The figure shows three views and two pictorial views of one solid part (mm, origin at its lowest corner). Answer the questions. A direction names the side the tool comes from. Give positions to 0.01 mm unless a question says otherwise; leave off trailing zeros. Loops run counter-clockwise (first coordinate to the right, second up) from the corner with the lowest first, then second, coordinate; pieces in that order, holes last. Notation, with made-up numbers: M -28,48 L 7,48 A35 ccw 7,87 Z; hole C 28.25,30.5 d10. An arc over 180 degrees is marked long. One line per item, written item: value. Start each with the question number.
Q1. The mould has two halves that part along Y. Classify the marked faces 1, 2 and 3: +Y half, -Y half, draft (parallel to the pull), parting line (faces both ways), or undercut.
Q2. A cutting plane is placed at A-A, the plane z = 8. Determine the outline of the cut face in (x, y), and give its area (4 significant figures).
Q3. A cutting plane is placed at D-D, the plane y = 13.25. Determine the outline of the cut face in (x, z).
Q4. A cutting plane is placed at B-B, the plane y = 9. Determine the outline of the cut face in (x, z), and give its area (4 significant figures).
Q5. For the marked faces 4 and 5, determine the directions among +Z, -Z, +X, -X, +Y, -Y from which every point of the face is accessible in a straight line to the end or side of a thin tool.
Q6. A cutting plane is placed at C-C, the plane x = 19.5. Determine the outline of the cut face in (y, z), and give its area (3 significant figures).
Q7. Flat-ended cylindrical pins translate along their axes: pin 1 (1.5 mm diameter, centred on x = 29, z = 11, fed in from -Y); pin 2 (4 mm diameter, centred on y = 4, z = 7, fed in from -X); pin 3 (6 mm diameter, centred on x = 22, z = 6.5, fed in from -Y); pin 4 (1 mm diameter, centred on y = 7.5, z = 1.5, fed in from +X). Find the tip coordinate at first contact, or state that the pin passes through.
Q8. Consider L1, parallel to Y at x = 17, z = 8; L2, parallel to X at y = 17, z = 0.5; L3, parallel to Y at x = 24, z = 3. Determine where each line is inside the solid, lowest interval first.
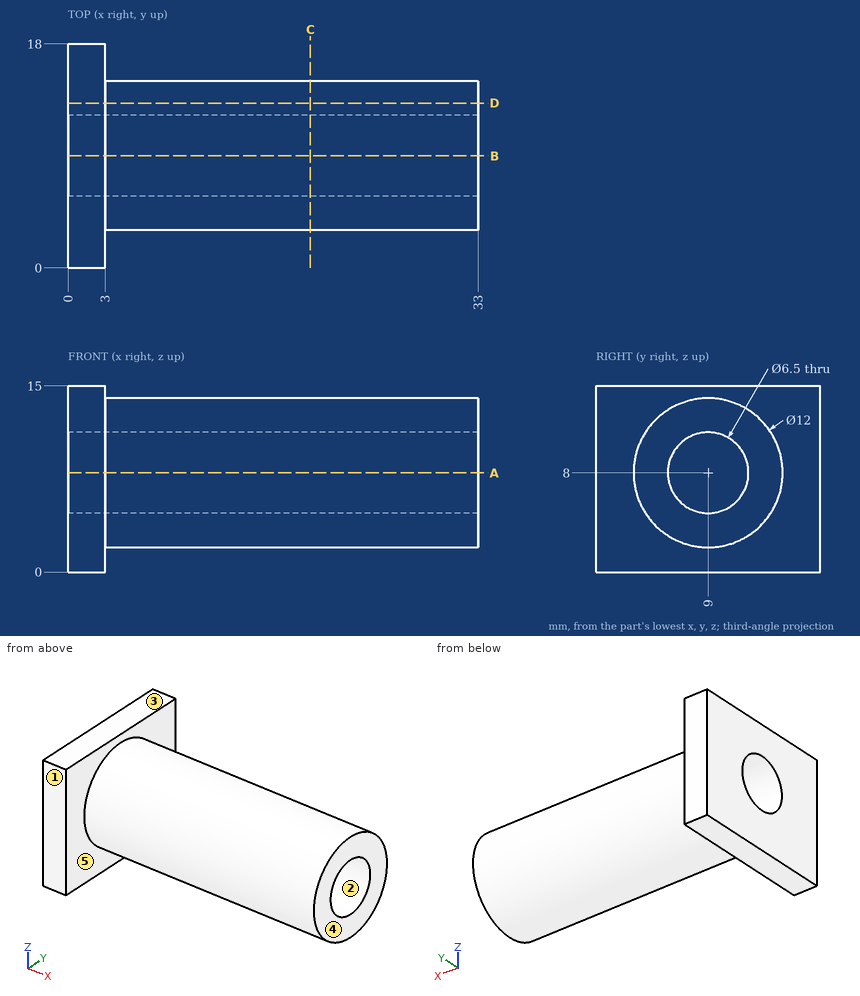
Answer block:
1. face 1: -Y half
1. face 2: undercut
1. face 3: draft
2. outline: M 0,0 L 3,0 L 3,3 L 33,3 L 33,5.75 L 0,5.75 Z; M 0,12.25 L 33,12.25 L 33,15 L 3,15 L 3,18 L 0,18 Z
2. area: 199.5 mm^2
3. outline: M 0,0 L 3,0 L 3,3.76 L 33,3.76 L 33,12.24 L 3,12.24 L 3,15 L 0,15 Z
4. outline: M 0,0 L 3,0 L 3,2 L 33,2 L 33,4.75 L 0,4.75 Z; M 0,11.25 L 33,11.25 L 33,14 L 3,14 L 3,15 L 0,15 Z
4. area: 190.5 mm^2
5. face 4: +Z, -Z, +X, +Y, -Y
5. face 5: +X
6. outline: C 9,8 d12; hole C 9,8 d6.5
6. area: 79.9 mm^2
7. pin 1: y = 3.44
7. pin 2: x = 0
7. pin 3: y = 3
7. pin 4: x = 3
8. L1: 3 to 5.75, 12.25 to 15
8. L2: 0 to 3
8. L3: 5.68 to 12.32
